Input: part model. Units: mm. Frame: model coordinates. Face numbers are marked on the shaded views. A direction names the side the tool comes from. Round coordinates to 2 decimals unless told otherwise and drop trailing zeros. Loops run counter-clockwise (first coordinate to the right, second up) from the corner with the lowest first, then second, coordinate; pieces in that order, holes last. Notation, with made-up numbers: (5, -8.75) -> (24, -8.75) arc R21 cw to (24, -4.75) -> close; hole circle Ø9 at (46, 27.5). An arc over 180 degrees is marked (long way). Answer as a JSON object with one key per item and string values. Group by question number.
Item 1: Section query A-A on z = 15.5. Return loops of the section in (x, y).
Item 2: Set-up query: the marked faces 5, 6, 7 and 8. Return all of +Z, -Z, +X, -X, +Y, -Y with unobstructed straight access to the full face (end or side cutting, diameter ignored); none if empty.
Item 3: Material intervals for line 1 (X direction, y = -4.5, z = 25); line 2 (X direction, y = -15, z = 28); line 3 (Y direction, x = -8, z = 41.5), sorted ascending. Write a range as [from, to].
Item 4: Section query C-C on y = -61. Return loops of the section in (x, z), and give its area (3 significant figures).
Item 5: Section query D-D on x = -9. Return loops of the section in (y, z).
Item 6: Draft query along X for the marked faces 1, 2, 3 and 4. Return one class per face: released by +X, released by -X, zero draft, split by the parting line, or undercut.
Item 7: Section query B-B on x = -33.5. Return loops of the section in (y, z), and give its area (3 significant figures).
Item 8: Pin query (flat end, axial travel): pin 1 (3 mm diameter, centred on x = -0.5, z = 10.5, fed in from +Y); pin 2 (3 mm diameter, centred on x = 1.5, y = -34.5, fed in from +Z) (3 decimals); pin 3 (8 mm diameter, centred on y = -65, z = 30.5, fed in from -X). Return the tip coordinate at first contact, or that it passes through.
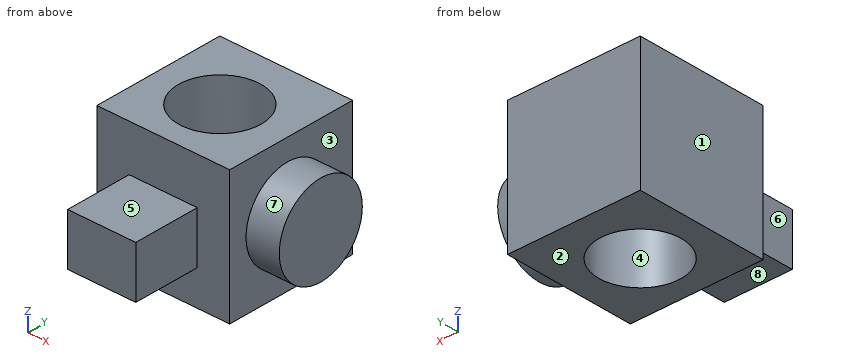
from build123d import *

# Parameters (mm, degrees)
F0_W     = 50.8
F0_H     = 50.8
F1_DEPTH = 50.8
F2_W     = 26.049768
F2_H     = 19.769912
F3_DEPTH = 25.4
F4_R     = 15.769687
F5_DEPTH = 50.8
F6_R     = 17.170546
F7_DEPTH = 12.7


with BuildPart() as f1:
    # F0 (on Front) → F1 (new body)
    with BuildSketch(Plane.XZ):
        with Locations((-27.746176, 25.4)):
            Rectangle(F0_W, F0_H)
    extrude(amount=F1_DEPTH)

    # F2 (on face) → F3 (join)
    with BuildSketch(Plane.XZ.offset(50.8)):
        with Locations((-27.794172, 23.258721)):
            Rectangle(F2_W, F2_H)
    extrude(amount=F3_DEPTH)

    # F4 (on face) → F5 (cut)
    with BuildSketch(Plane.XY.offset(50.8)):
        with Locations((-28.259346, -26.863825)):
            Circle(F4_R)
    extrude(amount=-F5_DEPTH, mode=Mode.SUBTRACT)

    # F6 (on face) → F7 (join)
    with BuildSketch(Plane.YZ.offset(-2.346176)):
        with Locations((-26.863823, 25.468299)):
            Circle(F6_R)
    extrude(amount=F7_DEPTH)


solid = f1.part
Solved:
{
 "1": {"outline": "(-53.15, -50.8) -> (-40.82, -50.8) -> (-40.82, -76.2) -> (-14.77, -76.2) -> (-14.77, -50.8) -> (-2.35, -50.8) -> (-2.35, -40.84) -> (10.35, -40.84) -> (10.35, -12.88) -> (-2.35, -12.88) -> (-2.35, 0) -> (-53.15, 0) -> close; hole circle Ø31.54 at (-28.26, -26.86)"},
 "2": {"face 5": "+Z, +X, -X, -Y", "face 6": "+Z, -Z, -X, -Y", "face 7": "+X", "face 8": "-Z, +X, -X, -Y"},
 "3": {"line 1": "[-53.15, -2.35]", "line 2": "[-53.15, -38.65], [-17.87, 10.35]", "line 3": "[-50.8, 0]"},
 "4": {"outline": "(-40.82, 13.37) -> (-14.77, 13.37) -> (-14.77, 33.14) -> (-40.82, 33.14) -> close", "area": "515 mm²"},
 "5": {"outline": "(-50.8, 0) -> (0, 0) -> (0, 50.8) -> (-50.8, 50.8) -> close"},
 "6": {"face 1": "released by -X", "face 2": "zero draft", "face 3": "released by +X", "face 4": "undercut"},
 "7": {"outline": "(-76.2, 13.37) -> (-50.8, 13.37) -> (-50.8, 0) -> (-41.74, 0) -> (-41.74, 50.8) -> (-50.8, 50.8) -> (-50.8, 33.14) -> (-76.2, 33.14) -> close; (-11.99, 0) -> (0, 0) -> (0, 50.8) -> (-11.99, 50.8) -> close", "area": "1,570 mm²"},
 "8": {"pin 1": "y = -16.21", "pin 2": "z = 41.505", "pin 3": "x = -40.82"}
}
